Work out the finished part from the listing and answer in its coordinate system (mm). Round coordinates to 2 decimals unless told otherwise and drop trailing zeros. Order: outer loops, then holes, each group sorted by start corner. A loop starts at its lowest first (then second) coordinate and runs counter-clockwise, first axis right, second up. Notation, with made-up numbers: (88.25, -35.5) -> (143.25, -35.5) arc R14 cw to (143.25, -25.5) -> close; hole circle Ø4 at (86, 12). An arc over 180 degrees is marked (long way). Use one line per item in the form item = value.
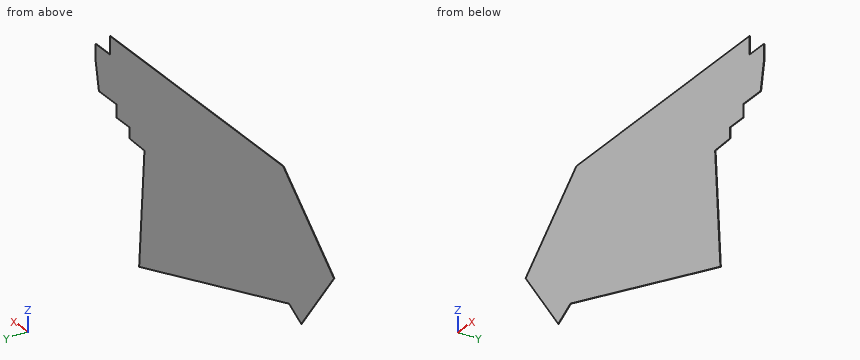
Autodesk Inventor part; units mm, degrees
ref_plane "YZ Plane" through (0, 0, 0) normal (1, 0, 0) x (0, 1, 0)
ref_plane "XZ Plane" through (0, 0, 0) normal (0, 1, 0) x (-1, 0, 0)
ref_plane "XY Plane" through (0, 0, 0) normal (0, 0, 1) x (1, 0, 0)
sketch "Sketch1" plane through (0, 0, 0) normal (0, 1, 0) x (-1, 0, 0)
  line L0 (0, 0) -> (620, 0)
  line L1 (620, 0) -> (802, -167)
  line L2 (802, -167) -> (685, -325)
  line L3 (685, -325) -> (641, -300)
  line L4 (641, -300) -> (104, -471)
  line L5 (104, -471) -> (123, -200)
  line L6 (123, -200) -> (70, -198)
  line L7 (70, -198) -> (70, -173)
  line L8 (70, -173) -> (22, -173)
  line L9 (22, -173) -> (22, -143)
  line L10 (22, -143) -> (-40, -143)
  line L11 (-40, -143) -> (-52, -80)
  line L12 (-52, -80) -> (-52, -42)
  line L13 (0, 0) -> (0, -42)
  line L14 (0, -42) -> (-52, -42)
  dimension "d0" = 620
  dimension "d1" = 802
  dimension "d2" = 167
  dimension "d3" = 685
  dimension "d4" = 325
  dimension "d5" = 641
  dimension "d6" = 300
  dimension "d7" = 104
  dimension "d8" = 471
  dimension "d9" = 123
  dimension "d10" = 200
  dimension "d11" = 70
  dimension "d12" = 198
  dimension "d13" = 173
  dimension "d14" = 22
  dimension "d15" = 143
  dimension "d16" = 40
  dimension "d17" = 80
  dimension "d18" = 52
  dimension "d19" = 42
extrude "Extrusion1" add sketch "Sketch1" along normal blind 1
properties part number "Contracted_profile"
Item 1: The part is cut by section A-A, the plane y = 0.35. Give the vertices of the cut face in (x, z).
Findings:
outline = (-802, -167) -> (-685, -325) -> (-641, -300) -> (-104, -471) -> (-123, -200) -> (-70, -198) -> (-70, -173) -> (-22, -173) -> (-22, -143) -> (40, -143) -> (52, -80) -> (52, -42) -> (0, -42) -> (0, 0) -> (-620, 0) -> close
Item 2: Flat-ended cylindrical pins translate along their axes: P1, Ø0.5, axis at x = 16, y = 0.5, coming from the +Z side; P2, Ø0.5, axis at x = -57, y = 0.5, coming from the -Z side. Find the tip coordinate at first contact, or state that the pin passes through.
Findings:
P1 = -42
P2 = -173
Item 3: The part is cut by section C-C, the plane z = -132. Give the vertices of the cut face in (x, y).
Findings:
outline = (-763.86, 0) -> (42.1, 0) -> (42.1, 1) -> (-763.86, 1) -> close
Item 4: Consider line 1 along Z through (x, y) = (-33, 0.45); line 2 along Z through (x, y) = (8, 0.1); line 3 along X through (y, z) = (0.8, -130). Determine where each line is inside the solid, lowest interval first.
Findings:
line_1 = -173 to 0
line_2 = -143 to -42
line_3 = -761.68 to 42.48
Item 5: The part is cut by section B-B, the plane x = -10. Give the vertices of the cut face in (y, z).
Findings:
outline = (0, -143) -> (1, -143) -> (1, 0) -> (0, 0) -> close
